Can you work these out from the model? Positions are in its coordinate system, mm. A direction names the side the tool comes from. Give positions to 0.01 mm unless a question says otherwise; leave off trailing zeros. Order: outer loops, then holes, each group sorted by start corner. A loop starts at its lowest first (then second) coordinate and runs counter-clockwise, first axis right, second up. Notation, with made-up numbers: M -12.5,18.25 L 31.5,18.25 A12 cw 31.5,40.25 Z; hole C 57,44.25 d9. An arc over 180 degrees is marked long. Answer as a JSON object with one key per item and string values.
```python
from build123d import *

# Parameters (mm, degrees)
BOSS_EXTRUDE1_DEPTH = 288.29
CUT_EXTRUDE2_REACH  = 301.942
SKETCH4_W           = 7.62
SKETCH4_H           = 23.8125
LPATTERN1_COUNT     = 3
LPATTERN1_PITCH     = 76.2


with BuildPart() as part:
    # Sketch1 → Boss-Extrude1 (new body)
    with BuildSketch(Plane.XY):
        Polygon((57.15, 0), (57.15, 31.75), (6.35, 31.75), (6.35, 0), (0, 0), (0, 31.75), (-10, 31.75), (-10, 38.1), (0, 38.1), (63.5, 38.1), (73.5, 38.1), (73.5, 31.75), (63.5, 31.75), (63.5, 9.525), (63.5, 0), align=None)
    extrude(amount=BOSS_EXTRUDE1_DEPTH)

    # Cut-Extrude2: up to this face of the body (flat: up to its plane)
    cut_extrude2_end = Plane(part.part.faces().sort_by_distance((0, 15.875, 144.145))[0])
    # Sketch4 → Cut-Extrude2 (cut, up to the picked face)
    with BuildSketch(Plane(origin=(63.5, 0, 0), x_dir=(0, 0, -1), z_dir=(1, 0, 0)), mode=Mode.PRIVATE) as cut_extrude2_sk1:
        with Locations((-220.345, 11.90625)):
            Rectangle(SKETCH4_W, SKETCH4_H)
    cut_extrude2_tool1 = split(extrude(cut_extrude2_sk1.sketch, amount=-CUT_EXTRUDE2_REACH, mode=Mode.PRIVATE), bisect_by=cut_extrude2_end, keep=Keep.BOTH, mode=Mode.PRIVATE)
    cut_extrude2 = cut_extrude2_tool1.solids().sort_by(Axis((63.5, 11.90625, 220.345), (-1, 0, 0)))[0]
    add(cut_extrude2, mode=Mode.SUBTRACT)

    # LPattern1: Cut-Extrude2 ×3
    with Locations(*[(0, 0, -i * LPATTERN1_PITCH) for i in range(1, LPATTERN1_COUNT)]):
        add(cut_extrude2, mode=Mode.SUBTRACT)


solid = part.part
```
1) Thinking about a two-plate mould opening in X: for faces 1 (the face through (0, 26, 142)), 2 (the face through (32, 31.75, 142)), 3 (the face through (60, 12, 140.335)), which applies, pulls with the +X half, pulls with the -X half, needs draft (parallel to the pull), parting line crosses it, or undercut?
Results found:
{"face 1": "pulls with the -X half", "face 2": "undercut", "face 3": "needs draft"}
2) I want a section at D-D on x = 60. Write out the boundary of the cut face in (y, z) (1 decimal).
Results found:
{"outline": "M 0,0 L 38.1,0 L 38.1,288.3 L 0,288.3 L 0,224.2 L 23.8,224.2 L 23.8,216.5 L 0,216.5 L 0,148 L 23.8,148 L 23.8,140.3 L 0,140.3 L 0,71.8 L 23.8,71.8 L 23.8,64.1 L 0,64.1 Z"}
3) I want a section at A-A on y = 28. Write out the boundary of the cut face in (x, z).
Results found:
{"outline": "M 0,0 L 6.35,0 L 6.35,288.29 L 0,288.29 Z; M 57.15,0 L 63.5,0 L 63.5,288.29 L 57.15,288.29 Z"}
4) I want a section at C-C on y = 16.5. Count the separate pieces of the cut face and the enclosed holes in it, and give its area (3 significant figures).
Results found:
{"separate pieces": "8", "enclosed holes": "0", "area": "3,370 mm²"}
5) For faces 4 (the face through (63.5, 26, 142)), 5 (the face through (3, 12, 216.535)), 6 (the face through (32, 38.1, 142)), 7 (the face through (6.35, 27, 142)), which set-ups out of +Z, -Z, +X, -X, +Y, -Y let a thin tool reach every point of the face, with its end or its side?
Results found:
{"face 4": "+Z, -Z, +X, -Y", "face 5": "+X, -X, -Y", "face 6": "+Z, -Z, +X, -X, +Y", "face 7": "+Z, -Z, -Y"}
6) I'm going to push flat-ended pins straight in: pin 1 Ø5 at (y, z) = (16.5, 44) entering from +X; pin 2 Ø4 at (x, z) = (14.5, 139.5) entering from -Y; pin 3 Ø5 at (x, z) = (4.5, 143) entering from -Y. Where does each tip first touch, or does it pass through?
Results found:
{"pin 1": "stops at x = 63.5", "pin 2": "stops at y = 31.75", "pin 3": "stops at y = 23.81"}
7) I want a section at B-B on z = 56.5. Write out the boundary of the cut face in (x, y).
Results found:
{"outline": "M -10,31.75 L 0,31.75 L 0,0 L 6.35,0 L 6.35,31.75 L 57.15,31.75 L 57.15,0 L 63.5,0 L 63.5,31.75 L 73.5,31.75 L 73.5,38.1 L -10,38.1 Z"}
8) I need wall thicknesses on L1, parallel to Z at x = 59.5, y = 19.5 (3 decimals); L2, parallel to X at y = 7, z = 62; L3, parallel to Y at x = 24.5, z = 57.5. Which ranges of each line are inside material? Lowest first, please.
Results found:
{"L1": "z = 0 to 64.135, 71.755 to 140.335, 147.955 to 216.535, 224.155 to 288.29", "L2": "x = 0 to 6.35, 57.15 to 63.5", "L3": "y = 31.75 to 38.1"}
